```python
from build123d import *

# Parameters (mm, degrees)
F0_W            = 22
F0_H            = 19
F1_DEPTH        = 3
F2_W            = 19
F2_H            = 3
F2_W_2          = 3
F2_H_2          = 19
F3_DEPTH        = 16
F5_D            = 4
F5_DEPTH        = 12
F5_CSINK_D      = 8
F5_CSINK_ANGLE  = 90
F5_TIP          = 1.2017212381
F7_D            = 4
F7_DEPTH        = 12
F7_CSINK_D      = 8
F7_CSINK_ANGLE  = 90
F7_TIP          = 1.2017212381
F9_D            = 4
F9_DEPTH        = 12
F9_CSINK_D      = 8
F9_CSINK_ANGLE  = 90
F9_TIP          = 1.2017212381
F11_D           = 4
F11_DEPTH       = 12
F11_CSINK_D     = 8
F11_CSINK_ANGLE = 90
F11_TIP         = 1.2017212381
F12_SIZE        = 0.75
F13_SIZE        = 0.75
F14_SIZE        = 0.75


with BuildPart() as f1:
    # F0 (on Top) → F1 (new body)
    with BuildSketch(Plane.XY):
        with Locations((30, -9.5)):
            Rectangle(F0_W, F0_H)
        with Locations((30, 31.5)):
            Rectangle(F0_W, F0_H)
        Polygon((0, 22), (0, 0), (19, 0), (41, 0), (60, 0), (60, 22), (41, 22), (19, 22), align=None)
    extrude(amount=F1_DEPTH)

    # F2 (on face) → F3 (join)
    with BuildSketch(Plane.XY.offset(3)):
        with Locations((9.5, 20.5)):
            Rectangle(F2_W, F2_H)
        Polygon((19, 41), (19, 22), (19, 19), (22, 19), (22, 41), align=None)
        with Locations((9.5, 1.5)):
            Rectangle(F2_W, F2_H)
        Polygon((19, 3), (19, 0), (19, -19), (22, -19), (22, 3), align=None)
        Polygon((60, 22), (41, 22), (38, 22), (38, 19), (60, 19), align=None)
        with Locations((39.5, 31.5)):
            Rectangle(F2_W_2, F2_H_2)
        with Locations((39.5, -9.5)):
            Rectangle(F2_W_2, F2_H_2)
        Polygon((38, 0), (41, 0), (60, 0), (60, 3), (38, 3), align=None)
    extrude(amount=F3_DEPTH)

    # F5
    with Locations(Plane.XZ):
        with Locations((9.5, 9.5)):
            CounterSinkHole(F5_D / 2, F5_CSINK_D / 2, depth=F5_DEPTH, counter_sink_angle=F5_CSINK_ANGLE)
            with Locations((0, 0, -(F5_DEPTH + F5_TIP / 2))):  # 118° drill point
                Cone(0, F5_D / 2, F5_TIP, mode=Mode.SUBTRACT)

    # F7
    with Locations(Plane.YZ.offset(41)):
        with Locations((-9.5, 9.5)):
            CounterSinkHole(F7_D / 2, F7_CSINK_D / 2, depth=F7_DEPTH, counter_sink_angle=F7_CSINK_ANGLE)
            with Locations((0, 0, -(F7_DEPTH + F7_TIP / 2))):  # 118° drill point
                Cone(0, F7_D / 2, F7_TIP, mode=Mode.SUBTRACT)

    # F9
    with Locations(Plane(origin=(0, 22, 0), x_dir=(-1, 0, 0), z_dir=(0, 1, 0))):
        with Locations((-50.5, 9.5)):
            CounterSinkHole(F9_D / 2, F9_CSINK_D / 2, depth=F9_DEPTH, counter_sink_angle=F9_CSINK_ANGLE)
            with Locations((0, 0, -(F9_DEPTH + F9_TIP / 2))):  # 118° drill point
                Cone(0, F9_D / 2, F9_TIP, mode=Mode.SUBTRACT)

    # F11
    with Locations(Plane(origin=(19, 0, 0), x_dir=(0, -1, 0), z_dir=(-1, 0, 0))):
        with Locations((-31.5, 9.5)):
            CounterSinkHole(F11_D / 2, F11_CSINK_D / 2, depth=F11_DEPTH, counter_sink_angle=F11_CSINK_ANGLE)
            with Locations((0, 0, -(F11_DEPTH + F11_TIP / 2))):  # 118° drill point
                Cone(0, F11_D / 2, F11_TIP, mode=Mode.SUBTRACT)

    # F12
    f12_edges = [f1.edges().sort_by_distance(p)[0] for p in [
        (19, -19, 9.5),
        (20.5, -19, 19),
        (22, -19, 11),
        (30, -19, 3),
        (38, -19, 11),
        (39.5, -19, 19),
        (41, -19, 9.5),
        (30, -19, 0),
        (60, 0, 9.5),
        (60, 1.5, 19),
        (60, 3, 11),
        (60, 11, 3),
        (60, 19, 11),
        (60, 20.5, 19),
        (60, 22, 9.5),
        (60, 11, 0),
        (41, 41, 9.5),
        (39.5, 41, 19),
        (38, 41, 11),
        (30, 41, 3),
        (22, 41, 11),
        (20.5, 41, 19),
        (19, 41, 9.5),
        (30, 41, 0),
        (0, 22, 9.5),
        (0, 20.5, 19),
        (0, 19, 11),
        (0, 11, 3),
        (0, 3, 11),
        (0, 1.5, 19),
        (0, 0, 9.5),
        (0, 11, 0),
    ]]
    chamfer(f12_edges, length=F12_SIZE)

    # F13
    f13_edges = [f1.edges().sort_by_distance(p)[0] for p in [
        (9.875, 22, 0),
        (19, 31.125, 0),
        (41, 31.125, 0),
        (50.125, 22, 0),
        (50.125, 0, 0),
        (41, -9.125, 0),
        (19, -9.125, 0),
        (9.875, 0, 0),
    ]]
    chamfer(f13_edges, length=F13_SIZE)

    # F14
    f14_edges = [f1.edges().sort_by_distance(p)[0] for p in [
        (50.125, 0, 19),
        (41, -9.125, 19),
        (38, -7.625, 19),
        (48.625, 3, 19),
        (38, 3, 11),
        (22, -7.625, 19),
        (19, -9.125, 19),
        (11.375, 3, 19),
        (22, 3, 11),
        (11.375, 19, 19),
        (9.875, 22, 19),
        (19, 31.125, 19),
        (22, 29.625, 19),
        (22, 19, 11),
        (48.625, 19, 19),
        (50.125, 22, 19),
        (41, 31.125, 19),
        (38, 29.625, 19),
        (38, 19, 11),
    ]]
    chamfer(f14_edges, length=F14_SIZE)


solid = f1.part
```
Check sheet for the modelled part. Datum: model origin and axes. Units: mm. A direction names the side the tool comes from. Round coordinates to 2 decimals unless told otherwise and drop trailing zeros. Loops run counter-clockwise (first coordinate to the right, second up) from the corner with the lowest first, then second, coordinate; pieces in that order, holes last. Notation, with made-up numbers: M 25.5,58 L 36.5,58 A19 cw 36.5,81 Z; hole C 55.5,88 d10. An arc over 180 degrees is marked long. Answer as a JSON object with one key per item and string values.
1. Section check C-C (z = 9.5). State how many separate pieces and enclosed holes the cut face has, plus the area to 3 significant figures.
Reply:
{"separate pieces": "8", "enclosed holes": "0", "area": "422 mm²"}
2. Access from +Z, -Z, +X, -X, +Y, -Y to the whole of each face (thin tool, end or side, straight path). Record for faces 4 (the flat face through (41, -9, 5)), 5 (the flat face through (50, 22, 5)), 6 (the flat face through (10, 22, 9)).
Reply:
{"face 4": "+Z, -Z, +X, -Y", "face 5": "+Z, -Z, +X, +Y", "face 6": "+Z, -Z, -X, +Y"}
3. Mould release check, pull along Z, two halves, no side actions. Record for faces 1 (the flat face through (14.7, 0.4, 19)), 2 (the flat face through (11, 19, 11)), 3 (the cylindrical face through (9.76, 2.507, 11.483)): pulls with the +Z half, pulls with the -Z half, needs draft (parallel to the pull), parting line crosses it, or undercut.
Reply:
{"face 1": "pulls with the +Z half", "face 2": "needs draft", "face 3": "undercut"}
4. Scan lines: line 1 (X direction, y = -16, z = 6.25); line 2 (Y direction, x = 21.3, z = 9.5); line 3 (Y direction, x = 16.5, z = 18). Record each from-to range of solid material in increasing order.
Reply:
{"line 1": "x = 19 to 22, 38 to 41", "line 2": "y = -18.95 to 2.95, 19.05 to 29.5, 33.5 to 40.95", "line 3": "y = 0 to 3, 19 to 22"}
5. Section check A-A (x = 50.5). Record the boundary of the cut face in (y, z), plus the area to 3 significant figures.
Reply:
{"outline": "M 0,0.75 L 0.75,0 L 21.25,0 L 22,0.75 L 22,5.5 L 20,7.5 L 19,7.5 L 19,3 L 3,3 L 3,18.25 L 2.25,19 L 0.75,19 L 0,18.25 Z; M 19,11.5 L 20,11.5 L 22,13.5 L 22,18.25 L 21.25,19 L 19.75,19 L 19,18.25 Z", "area": "144 mm²"}
6. Gauge pin test, flat ends, axial feed: P1, Ø8, axis at x = 32, y = 28, coming from the +Z side; P2, Ø6.5, axis at y = -9.5, z = 9.5, coming from the +X side; P3, Ø1.5, axis at y = -5.5, z = 2.5, coming from the -X side. Record the tip position at first contact, or that the pin passes through.
Reply:
{"P1": "stops at z = 3", "P2": "stops at x = 40.25", "P3": "stops at x = 19"}
7. Section check B-B (y = 15). Record the boundary of the cut face in (x, z), plus the area to 3 significant figures.
Reply:
{"outline": "M 0,0.75 L 0.75,0 L 59.25,0 L 60,0.75 L 60,2.25 L 59.25,3 L 0.75,3 L 0,2.25 Z", "area": "179 mm²"}
8. Section check D-D (x = 34). Record the boundary of the cut face in (y, z), plus the area to 3 significant figures.
Reply:
{"outline": "M -19,0.75 L -18.25,0 L 40.25,0 L 41,0.75 L 41,2.25 L 40.25,3 L -18.25,3 L -19,2.25 Z", "area": "179 mm²"}
